The listing builds one solid part. Answer for the finished solid, in the listing's coordinates (mm). Face numbers are marked on the shaded views. A direction names the side the tool comes from. Give positions to 0.01 mm unless a question says otherwise; leave off trailing zeros. Order: outer loops, then holes, each group sorted by start corner. A loop starts at its lowest first (then second) coordinate and runs counter-clockwise, first axis right, second up. Notation, with made-up numbers: (-17.5, 56.5) - (11.5, 56.5) arc R22 ccw to (11.5, 73.5) - close; hole circle Ø6 at (10.25, 54.25). An arc over 180 degrees is marked (long way). Answer as CSV lines item,"result". Start each with the question number.
1. Consider line 1 along Y through (x, z) = (-4.75, 1.75); line 2 along Z through (x, y) = (-0.5, 2.5); line 3 along X through (y, z) = (-0.5, 3.5). Determine where each line is inside the solid, lowest interval first. Write a range as [from, to].
2. Section D-D on z = -2.25 is taken. Give the vertices of the cut face in (x, y).
3. Flat-ended cylindrical pins translate along their axes: pin 1 (0.6 mm diameter, centred on x = 4.5, z = -1, fed in from +Y); pin 2 (2 mm diameter, centred on x = -1, y = -0.5, fed in from -Z). Find the tip coordinate at first contact, or state that the pin passes through.
4. Section A-A on y = -0.45 is taken. Give the vertices of the cut face in (x, z), and give its area (3 significant figures).
5. Section B-B on z = 0 is taken. Give the vertices of the cut face in (x, y).
6. Which of the six approach directions +Z, -Z, +X, -X, +Y, -Y give full straight-line access (tool end or side, diameter ignored) to the marked faces 1, 2, 3, 4 and 5?
7. Section C-C on x = -3.95 is taken. Give the vertices of the cut face in (y, z), and give its area (3 significant figures).
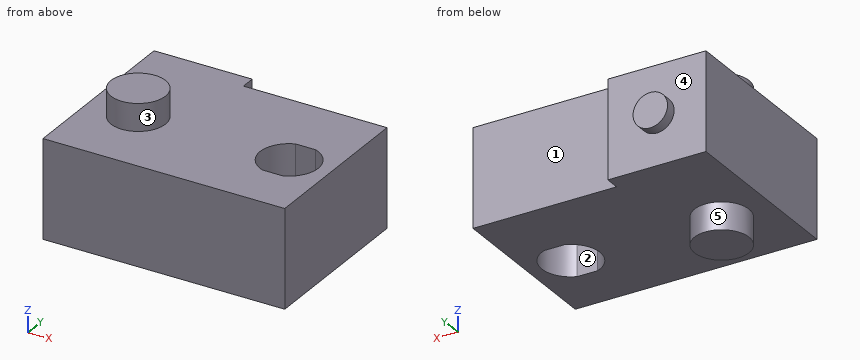
from build123d import *

# Parameters (mm, degrees)
BOSS_EXTRUDE1_DEPTH      = 2.7
BOSS_EXTRUDE2_DEPTH      = 4.2
BOSS_EXTRUDE2_DEPTH_BACK = 4.2
SKETCH3_R                = 1.5
SKETCH4_R                = 0.95
BOSS_EXTRUDE3_DEPTH      = 0.6


with BuildPart() as part:
    # Sketch1 → Boss-Extrude1 (new, symmetric)
    with BuildSketch(Plane.XY):
        Polygon((6.65, -4.65), (-6.65, -4.65), (-6.65, 4.65), (-6.65, 5.45), (-1.25, 5.45), (-1.25, 4.65), (6.65, 4.65), align=None)
        with BuildLine():
            Line((3.793223564, 1.05), (4.906776436, 1.05))
            ThreePointArc((4.906776436, 1.05), (5.95, -0.45), (4.906776436, -1.95))
            Line((4.906776436, -1.95), (3.793223564, -1.95))
            ThreePointArc((3.793223564, -1.95), (2.75, -0.45), (3.793223564, 1.05))
        make_face(mode=Mode.SUBTRACT)
    extrude(amount=BOSS_EXTRUDE1_DEPTH, both=True)

    # Sketch3 → Boss-Extrude2 (add, two sides: drawn at the far end of the back side and taken through both)
    with BuildSketch(Plane.XY.offset(-BOSS_EXTRUDE2_DEPTH_BACK)):
        with Locations(Location((-3.95, -0.45, 0), (0, 0, 180))):
            Circle(SKETCH3_R)
    extrude(amount=BOSS_EXTRUDE2_DEPTH + BOSS_EXTRUDE2_DEPTH_BACK)

    # Sketch4 → Boss-Extrude3 (add)
    with BuildSketch(Plane(origin=(0, 5.45, 0), x_dir=(1, 0, 0), z_dir=(0, 1, 0))):
        with Locations(Location((-3.95, 0, 0), (0, 0, 180))):
            Circle(SKETCH4_R)
    extrude(amount=BOSS_EXTRUDE3_DEPTH)


solid = part.part
Checks:
1,line 1,"y = [-4.65, 5.45]"
1,line 2,"z = [-2.7, 2.7]"
1,line 3,"x = [-5.45, -2.45]"
2,outline,"(-6.65, -4.65) - (6.65, -4.65) - (6.65, 4.65) - (-1.25, 4.65) - (-1.25, 5.45) - (-6.65, 5.45) - close; hole (3.79, -1.95) - (4.91, -1.95) arc R1.6 ccw to (4.91, 1.05) - (3.79, 1.05) arc R1.6 ccw to start"
3,pin 1,"stops at y = 4.65"
3,pin 2,"stops at z = -2.7"
4,outline,"(-6.65, -2.7) - (-5.45, -2.7) - (-5.45, -4.2) - (-2.45, -4.2) - (-2.45, -2.7) - (2.75, -2.7) - (2.75, 2.7) - (-2.45, 2.7) - (-2.45, 4.2) - (-5.45, 4.2) - (-5.45, 2.7) - (-6.65, 2.7) - close; (5.95, -2.7) - (6.65, -2.7) - (6.65, 2.7) - (5.95, 2.7) - close"
4,area,"63.5 mm²"
5,outline,"(-6.65, -4.65) - (6.65, -4.65) - (6.65, 4.65) - (-1.25, 4.65) - (-1.25, 5.45) - (-3, 5.45) - (-3, 6.05) - (-4.9, 6.05) - (-4.9, 5.45) - (-6.65, 5.45) - close; hole (3.79, -1.95) - (4.91, -1.95) arc R1.6 ccw to (4.91, 1.05) - (3.79, 1.05) arc R1.6 ccw to start"
6,face 1,"+Z, -Z, +X, +Y"
6,face 2,"+Z, -Z"
6,face 3,"+Z"
6,face 4,"+Y"
6,face 5,"-Z"
7,outline,"(-4.65, -2.7) - (-1.95, -2.7) - (-1.95, -4.2) - (1.05, -4.2) - (1.05, -2.7) - (5.45, -2.7) - (5.45, -0.95) - (6.05, -0.95) - (6.05, 0.95) - (5.45, 0.95) - (5.45, 2.7) - (1.05, 2.7) - (1.05, 4.2) - (-1.95, 4.2) - (-1.95, 2.7) - (-4.65, 2.7) - close"
7,area,"64.7 mm²"
